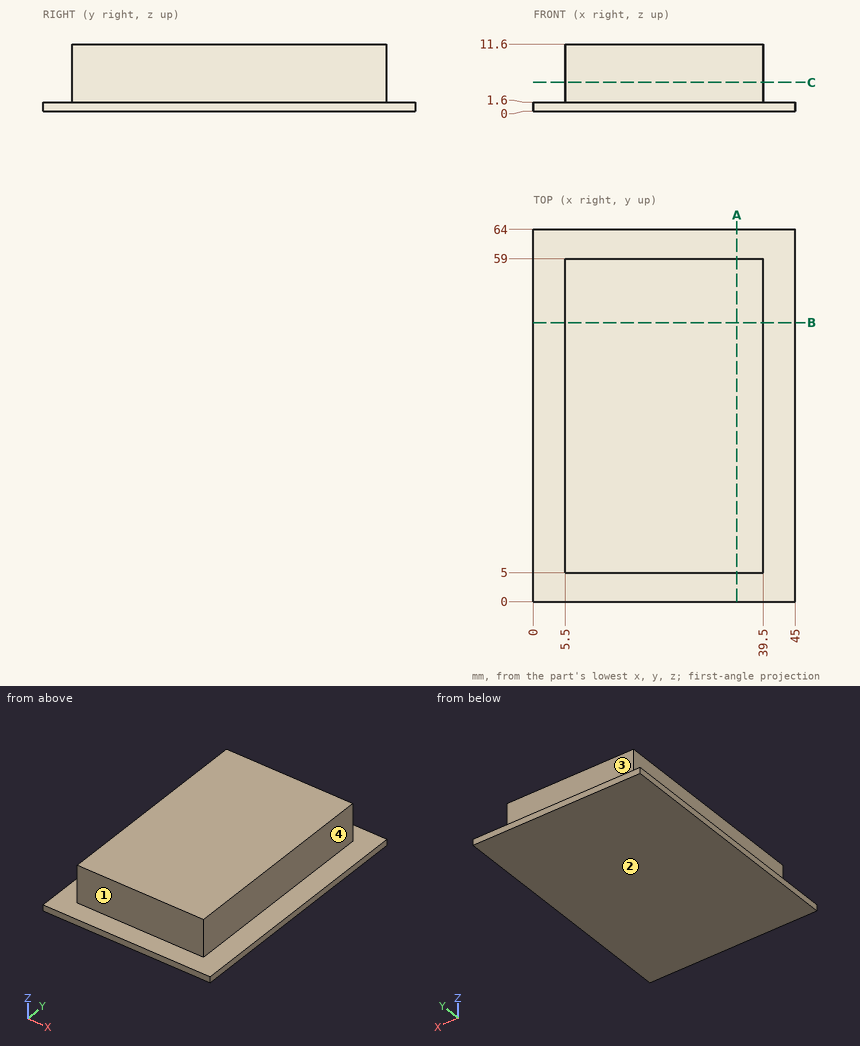
The drawing under review shows one solid part. Ordinate dimensions are in mm from its lowest x, y, z. A direction names the side the tool comes from. Coordinates: 2 decimals unless noted, no trailing zeros. Loops run counter-clockwise (first coordinate to the right, second up) from the corner with the lowest first, then second, coordinate; pieces in that order, holes last. Notation, with made-up numbers: (43.25, 67.25) - (50.25, 67.25) arc R25 ccw to (50.25, 81.25) - close; hole circle Ø11 at (-21.5, 15). An arc over 180 degrees is marked (long way). Return JSON: item names as keys, results as strings.
Item 1: Take a section at B-B (y = 48). Give the boundary of the cut face in (x, z).
Determined:
{"outline": "(0, 0) - (45, 0) - (45, 1.6) - (39.5, 1.6) - (39.5, 11.6) - (5.5, 11.6) - (5.5, 1.6) - (0, 1.6) - close"}
Item 2: For the marked faces 1, 2, 3 and 4, list the 3-axis set-ups (+Z, -Z, +X, -X, +Y, -Y) from which the entire face can be reached by the end or side of a thin tool; tool diameter is ignored.
Determined:
{"face 1": "+Z, +X, -X, -Y", "face 2": "-Z, +X, -X, +Y, -Y", "face 3": "+Z, +X, -X, +Y", "face 4": "+Z, +X, +Y, -Y"}
Item 3: Take a section at A-A (x = 35). Give the boundary of the cut face in (y, z), then the cut area to 3 significant figures.
Determined:
{"outline": "(0, 0) - (64, 0) - (64, 1.6) - (59, 1.6) - (59, 11.6) - (5, 11.6) - (5, 1.6) - (0, 1.6) - close", "area": "642 mm2"}
Item 4: For line 1 (Y direction, x = 31.5, z = 8.5); line 2 (X direction, y = 22.5, z = 4); line 3 (Z direction, x = 35, y = 3), list the stretches that pass through material, from the lowest coordinate up.
Determined:
{"line 1": "y = 5 to 59", "line 2": "x = 5.5 to 39.5", "line 3": "z = 0 to 1.6"}
Item 5: Insertion check: pin 1 (3 mm diameter, centred on x = 23, z = 8, fed in from +Y); pin 2 (2 mm diameter, centred on y = 33.5, z = 3, fed in from -X); pin 3 (5 mm diameter, centred on y = 35, z = 8, fed in from +X). Each pin has a flat end and moves straight along its axis. Give the tip position at first contact, or say it passes through.
Determined:
{"pin 1": "stops at y = 59", "pin 2": "stops at x = 5.5", "pin 3": "stops at x = 39.5"}
Item 6: Take a section at C-C (z = 5). Give the boundary of the cut face in (x, y).
Determined:
{"outline": "(5.5, 5) - (39.5, 5) - (39.5, 59) - (5.5, 59) - close"}
